Verification items for the finished model (mm, model axes). A direction names the side the tool comes from. Give positions to 0.01 mm unless a question says otherwise; leave off trailing zeros. Write each loop counter-clockwise with the first axis right and the second up, starting at its lowest first coordinate (ties: lowest second). Pieces come first, ordered by that corner, then holes. Notation, with made-up numbers: M -26,31.25 L -12,31.25 A19 ccw -12,58.25 Z; hole C 76.25,-22.5 d5. An arc over 180 degrees is marked long. Write item = value, one per line.
from build123d import *

# Parameters (mm, degrees)
SKETCH1_W           = 48
SKETCH1_H           = 24
BOSS_EXTRUDE1_DEPTH = 34
SHELL1_T            = -2
CUT_EXTRUDE1_DEPTH  = 2
SKETCH3_W           = 6.5
SKETCH3_H           = 17.142463893
BOSS_EXTRUDE2_DEPTH = 32
SKETCH4_R           = 1.75
CUT_EXTRUDE2_DEPTH  = 10


with BuildPart() as part:
    # Sketch1 → Boss-Extrude1 (new body)
    with BuildSketch(Plane(origin=(0, 0, 0), x_dir=(1, 0, 0), z_dir=(0, 1, 0))):
        with Locations((0, -2.545302013)):
            Rectangle(SKETCH1_W, SKETCH1_H)
    extrude(amount=BOSS_EXTRUDE1_DEPTH)

    # Shell1
    shell1_openings = [part.faces().sort_by_distance(p)[0] for p in [
        (0, 0, 2.545302013),
    ]]
    offset(amount=SHELL1_T, openings=shell1_openings, kind=Kind.INTERSECTION)

    # Sketch2 → Cut-Extrude1 (cut)
    with BuildSketch(Plane(origin=(0, 0, -9.454697987), x_dir=(-1, 0, 0), z_dir=(0, 0, -1))):
        with BuildLine():
            Line((-6.502577746, 0), (6.502577746, 0))
            Line((6.502577746, 0), (6.502577746, 25))
            ThreePointArc((6.502577746, 25), (0, 31.502577746), (-6.502577746, 25))
            Line((-6.502577746, 25), (-6.502577746, 0))
        make_face()
    extrude(amount=-CUT_EXTRUDE1_DEPTH, mode=Mode.SUBTRACT)

    # Sketch3 → Boss-Extrude2 (add)
    with BuildSketch(Plane.XZ.offset(-32)):
        with Locations((18.75, 3.974070066)):
            Rectangle(SKETCH3_W, SKETCH3_H)
        with Locations((-18.75, 3.974070066)):
            Rectangle(SKETCH3_W, SKETCH3_H)
    extrude(amount=BOSS_EXTRUDE2_DEPTH)

    # Sketch4 → Cut-Extrude2 (cut)
    with BuildSketch(Plane.XZ):
        with Locations((20, 5.545302013)):
            Circle(SKETCH4_R)
        with Locations((-20, 5.545302013)):
            Circle(SKETCH4_R)
    extrude(amount=-CUT_EXTRUDE2_DEPTH, mode=Mode.SUBTRACT)


solid = part.part
1) Cross-section at A-A on x = 0. Record the boundary of the cut face in (y, z), plus the area to 3 significant figures.
From the geometry:
outline = M 0,12.55 L 32,12.55 L 32,-7.45 L 31.5,-7.45 L 31.5,-9.45 L 34,-9.45 L 34,14.55 L 0,14.55 Z
area = 113 mm^2
2) Cross-section at D-D on y = 16. Record the boundary of the cut face in (x, z).
From the geometry:
outline = M -24,-9.45 L -6.5,-9.45 L -6.5,-7.45 L -22,-7.45 L -22,-4.6 L -15.5,-4.6 L -15.5,12.55 L 15.5,12.55 L 15.5,-4.6 L 22,-4.6 L 22,-7.45 L 6.5,-7.45 L 6.5,-9.45 L 24,-9.45 L 24,14.55 L -24,14.55 Z
3) Depth check by flat-ended pin: P1, Ø1, axis at x = -20, z = 6, coming from the -Y side. Enter the tip coordinate at first touch or a pass-through.
From the geometry:
P1 = 10
4) Draft check along Z on faces 4 (the flat face through (10, 17, -9.455)), 5 (the flat face through (-10, 16, -7.455)), 6 (the flat face through (0, 34, 2)). Enter one of: +Z half, -Z half, draft (parallel to the pull), parting line (faces both ways), or undercut.
From the geometry:
face_4 = -Z half
face_5 = undercut
face_6 = draft
5) Cross-section at B-B on y = 2. Record the boundary of the cut face in (x, z).
From the geometry:
outline = M -24,-9.45 L -6.5,-9.45 L -6.5,-7.45 L -22,-7.45 L -22,-4.6 L -15.5,-4.6 L -15.5,12.55 L 15.5,12.55 L 15.5,-4.6 L 22,-4.6 L 22,-7.45 L 6.5,-7.45 L 6.5,-9.45 L 24,-9.45 L 24,14.55 L -24,14.55 Z; hole C -20,5.55 d3.5; hole C 20,5.55 d3.5
6) Material ranges on probe 1 along Z at (x, y) = (20, 5); probe 2 along X at (y, z) = (23, 3); probe 3 along Z at (x, y) = (11, 4.5), recorded low to high. Write a range as from..to.
From the geometry:
probe_1 = -9.45..-7.45, -4.6..3.8, 7.3..14.55
probe_2 = -24..-15.5, 15.5..24
probe_3 = -9.45..-7.45, 12.55..14.55
7) Tool access check on faces 1 (the cylindrical face through (-21.29, 4.93, 6.73)), 2 (the flat face through (-24, 17, 3)), 3 (the flat face through (6.503, 13, -8)). Record the directions out of +Z, -Z, +X, -X, +Y, -Y that give a thin tool (end or side, any length) a straight path to the whole face; none if there is none.
From the geometry:
face_1 = -Y
face_2 = +Z, -Z, -X, +Y, -Y
face_3 = -Z, -Y
8) Cross-section at C-C on z = 1.25. Record the boundary of the cut face in (x, y), plus the area to 3 significant figures.
From the geometry:
outline = M -24,0 L -15.5,0 L -15.5,32 L 15.5,32 L 15.5,0 L 24,0 L 24,34 L -24,34 Z
area = 640 mm^2
